Can you work these out from the model? Positions are in its coordinate system, mm. A direction names the side the tool comes from. Round coordinates to 2 decimals unless told otherwise and drop trailing zeros. Write each loop counter-clockwise with the first axis right and the second up, starting at its lowest first coordinate (ties: lowest second). Pieces come first, ordered by that corner, then holes. Notation, with made-up numbers: (28, -23) -> (61, -23) arc R22 cw to (61, 15) -> close; hole circle Ø10 at (37.5, 88.25). An arc over 180 degrees is marked (long way). Use CSV: the item, a comma, the result in double quotes.
```python
from build123d import *

# Parameters (mm, degrees)
SKETCH1_R               = 1.7
BOSS_EXTRUDE1_DEPTH     = 2
CUT_EXTRUDE1_DEPTH      = 1
CUT_EXTRUDE1_DEPTH_BACK = 3


with BuildPart() as part:
    # Sketch1 → Boss-Extrude1 (new body)
    with BuildSketch(Plane.XY):
        with BuildLine():
            ThreePointArc((-29.5, 16.4), (-31.550609665, 15.550609665), (-32.4, 13.5))
            Line((-32.4, 13.5), (-32.4, -10.5))
            ThreePointArc((-32.4, -10.5), (-31.550609665, -12.550609665), (-29.5, -13.4))
            Line((-29.5, -13.4), (-5.5, -13.4))
            ThreePointArc((-5.5, -13.4), (-3.449390335, -12.550609665), (-2.6, -10.5))
            Line((-2.6, -10.5), (-2.6, 13.5))
            ThreePointArc((-2.6, 13.5), (-3.449390335, 15.550609665), (-5.5, 16.4))
            Line((-5.5, 16.4), (-29.5, 16.4))
        make_face()
        with Locations((-29.5, -10.5)):
            Circle(SKETCH1_R, mode=Mode.SUBTRACT)
        with Locations((-5.5, -10.5)):
            Circle(SKETCH1_R, mode=Mode.SUBTRACT)
        with Locations((-29.5, 13.5)):
            Circle(SKETCH1_R, mode=Mode.SUBTRACT)
        with Locations((-5.5, 13.5)):
            Circle(SKETCH1_R, mode=Mode.SUBTRACT)
    extrude(amount=-BOSS_EXTRUDE1_DEPTH)

    # Sketch3 → Cut-Extrude1 (cut, two sides)
    with BuildSketch(Plane.XY) as cut_extrude1_sk:
        with BuildLine():
            Line((-23.75, 10.5), (-11.25, 10.5))
            ThreePointArc((-11.25, 10.5), (-10, 9.25), (-11.25, 8))
            Line((-11.25, 8), (-23.75, 8))
            ThreePointArc((-23.75, 8), (-25, 9.25), (-23.75, 10.5))
        make_face()
        with BuildLine():
            Line((-26.25, 6), (-8.75, 6))
            ThreePointArc((-8.75, 6), (-7, 4.25), (-8.75, 2.5))
            Line((-8.75, 2.5), (-26.25, 2.5))
            ThreePointArc((-26.25, 2.5), (-28, 4.25), (-26.25, 6))
        make_face()
        with BuildLine():
            Line((-26.25, -3), (-8.75, -3))
            ThreePointArc((-8.75, -3), (-7, -1.25), (-8.75, 0.5))
            Line((-8.75, 0.5), (-26.25, 0.5))
            ThreePointArc((-26.25, 0.5), (-28, -1.25), (-26.25, -3))
        make_face()
        with BuildLine():
            Line((-23.75, -7.5), (-11.25, -7.5))
            ThreePointArc((-11.25, -7.5), (-10, -6.25), (-11.25, -5))
            Line((-11.25, -5), (-23.75, -5))
            ThreePointArc((-23.75, -5), (-25, -6.25), (-23.75, -7.5))
        make_face()
    extrude(amount=CUT_EXTRUDE1_DEPTH, mode=Mode.SUBTRACT)
    extrude(cut_extrude1_sk.sketch, amount=-CUT_EXTRUDE1_DEPTH_BACK, mode=Mode.SUBTRACT)


solid = part.part
```
Q1. Suppose I cut it at A-A (y = -6.25). Write out the boundary of the cut face in (x, z).
Resolved:
outline,"(-32.4, -2) -> (-25, -2) -> (-25, 0) -> (-32.4, 0) -> close; (-10, -2) -> (-2.6, -2) -> (-2.6, 0) -> (-10, 0) -> close"
Q2. On a 3-axis mill with a long thin cutter (end or side, diameter ignored), from which of +Z, -Z, +X, -X, +Y, -Y can I reach the whole of each face in a straight line? I mean faces 4 (the face through (-3.4, 15.5, -1)), 5 (the face through (-28, -1.2, -1)). Say none if no direction works.
Resolved:
face 4,"+Z, -Z, +X, +Y"
face 5,"+Z, -Z"
Q3. Suppose I cut it at D-D (y = -11.5). Write out the boundary of the cut face in (x, z), and give its area (3 significant figures).
Resolved:
outline,"(-32.22, -2) -> (-30.87, -2) -> (-30.87, 0) -> (-32.22, 0) -> close; (-28.13, -2) -> (-6.87, -2) -> (-6.87, 0) -> (-28.13, 0) -> close; (-4.13, -2) -> (-2.78, -2) -> (-2.78, 0) -> (-4.13, 0) -> close"
area,"47.9 mm^2"
Q4. Please list where these lines run through material, in increasing order: probe 1 along Y at (x, z) = (-22, -1); probe 2 along Y at (x, z) = (-29.5, -0.35); probe 3 along Y at (x, z) = (-9.5, -0.9).
Resolved:
probe 1,"y = -13.4 to -7.5, -5 to -3, 0.5 to 2.5, 6 to 8, 10.5 to 16.4"
probe 2,"y = -13.4 to -12.2, -8.8 to 11.8, 15.2 to 16.4"
probe 3,"y = -13.4 to -3, 0.5 to 2.5, 6 to 16.4"
Q5. Suppose I cut it at C-C (z = -1). Count the separate pieces of the cut face and the enclosed holes in it, and give its area (3 significant figures).
Resolved:
separate pieces,"1"
enclosed holes,"8"
area,"630 mm^2"
Q6. If we mould it in two halves opening along X, with no side actions, what happens to faces 1 (the face through (-25, 9.2, -1)), 2 (the face through (-31.6, -12.5, -1)), 3 (the face through (-2.6, 1, -1))? For each: released by +X, released by -X, zero draft, split by the parting line, or undercut.
Resolved:
face 1,"undercut"
face 2,"released by -X"
face 3,"released by +X"
Q7. Suppose I cut it at B-B (x = -17). Write out the boundary of the cut face in (y, z), and give its area (3 significant figures).
Resolved:
outline,"(-13.4, -2) -> (-7.5, -2) -> (-7.5, 0) -> (-13.4, 0) -> close; (-5, -2) -> (-3, -2) -> (-3, 0) -> (-5, 0) -> close; (0.5, -2) -> (2.5, -2) -> (2.5, 0) -> (0.5, 0) -> close; (6, -2) -> (8, -2) -> (8, 0) -> (6, 0) -> close; (10.5, -2) -> (16.4, -2) -> (16.4, 0) -> (10.5, 0) -> close"
area,"35.6 mm^2"
